Job drawing, mm, ordinate dimensions from the low corner. One solid piece. Give positions to 0.01 mm unless a question says otherwise; leave off trailing zeros. Order: outer loops, then holes, each group sorted by start corner. A loop starts at its lowest first (then second) coordinate and runs counter-clockwise, first axis right, second up.
1. Slice it at A-A on x = 10.55. List the corners of the cut face in (y, z).
2. Slice it at D-D on x = 17. List the corners of the cut face in (y, z) (1 decimal), and give its area (3 significant figures).
3. Probe line 1 (Z direction, x = 10.55, y = 6); line 2 (X direction, y = 6.75, z = 8.25) (1 decimal); line 3 (X direction, y = 9, z = 5) (1 decimal). List the from-to ranges inside material, lowest first.
4. Drop flat-ended pins along their axis: pin 1 Ø1.5 at (y, z) = (5, 7.5) entering from -X; pin 2 Ø5 at (y, z) = (8.5, 15) entering from +X; pin 3 Ø1.5 at (x, z) = (7.5, 14) entering from +Y. Give the stop position or say it passes through.
5. Slice it at C-C on z = 5.25. List the corners of the cut face in (x, y), and give its area (3 significant figures).
6. Mould opens along X. For the marked faces 1, 2 and 3 say: +X half, -X half, draft (parallel to the pull), parting line (faces both ways), or undercut.
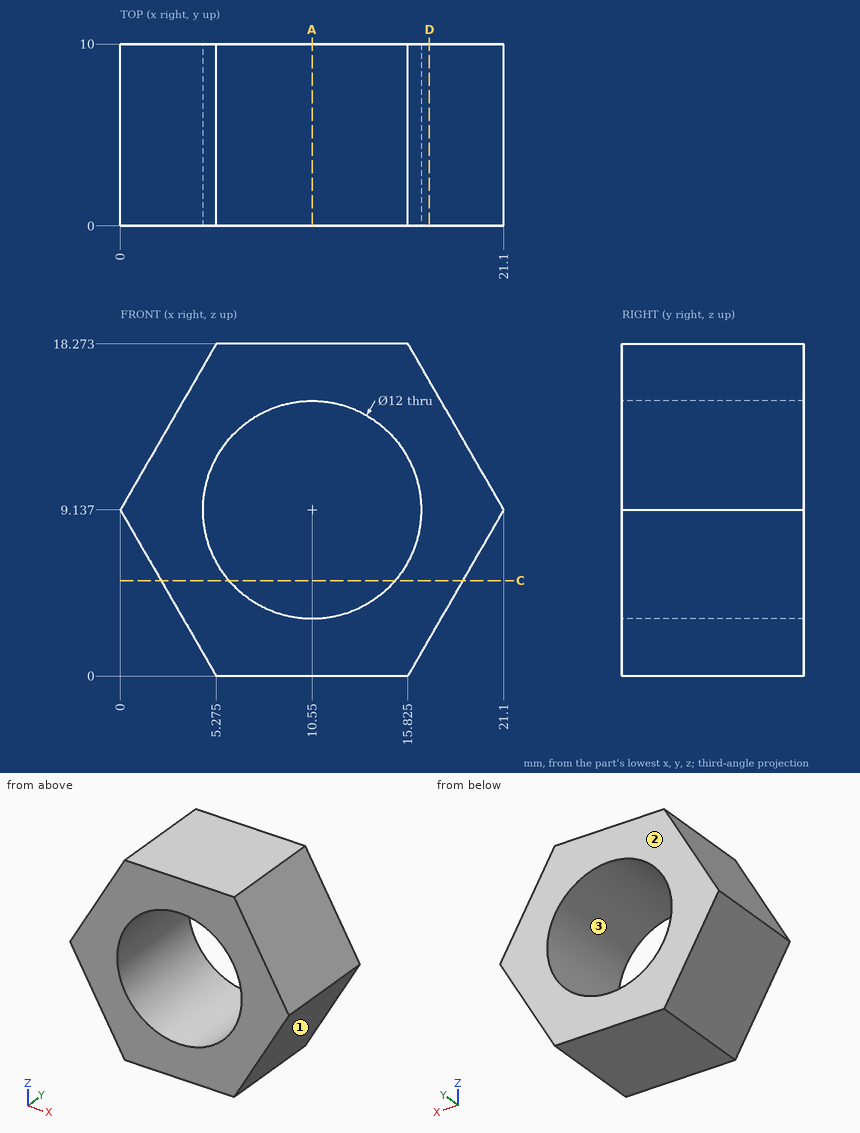
Data:
1. outline: (0, 0) - (10, 0) - (10, 3.14) - (0, 3.14) - close; (0, 15.14) - (10, 15.14) - (10, 18.27) - (0, 18.27) - close
2. outline: (0, 2) - (10, 2) - (10, 16.2) - (0, 16.2) - close
2. area: 142 mm2
3. line 1: z = 0 to 3.14, 15.14 to 18.27
3. line 2: x = 0.5 to 4.6, 16.5 to 20.6
3. line 3: x = 2.4 to 6.2, 14.9 to 18.7
4. pin 1: stops at x = 0.51
4. pin 2: stops at x = 19.16
4. pin 3: stops at y = 10
5. outline: (2.24, 0) - (5.98, 0) - (5.98, 10) - (2.24, 10) - close; (15.12, 0) - (18.86, 0) - (18.86, 10) - (15.12, 10) - close
5. area: 74.7 mm2
6. face 1: +X half
6. face 2: draft
6. face 3: undercut
